Read the model definition and answer for the solid it produces. Units are mm, in the model's axes. A direction names the side the tool comes from. Give positions to 0.01 mm unless a question says otherwise; leave off trailing zeros. Loops run counter-clockwise (first coordinate to the right, second up) from the corner with the lowest first, then second, coordinate; pieces in that order, holes last. Notation, with made-up numbers: (-28, 60) -> (-20, 60) arc R24 cw to (-20, 75) -> close; hole circle Ø9 at (-6, 64.5). An arc over 180 degrees is marked (long way). One line per item, written item: value. Start each with the question number.
from build123d import *

# Parameters (mm, degrees)
SZKIC1_W                    = 33
SZKIC1_H                    = 20
DODANIE_WYCI_GNI_CIE1_DEPTH = 6
SZKIC2_W                    = 9.7
SZKIC2_H                    = 16
WYTNIJ_WYCI_GNI_CIE1_DEPTH  = 5
SZKIC2_4_W                  = 6.5
SZKIC2_4_H                  = 16
WYTNIJ_WYCI_GNI_CIE2_DEPTH  = 21.205197351
SZKIC3_W                    = 15.9
SZKIC3_H                    = 27
DODANIE_WYCI_GNI_CIE2_DEPTH = 4
SZKIC4_W                    = 10.5
SZKIC4_H                    = 23.5
WYTNIJ_WYCI_GNI_CIE3_DEPTH  = 2.5


with BuildPart() as part:
    # Szkic1 → Dodanie-wyciągnięcie1 (new body)
    with BuildSketch(Plane(origin=(0, 0, 0), x_dir=(1, 0, 0), z_dir=(0, 1, 0))):
        Rectangle(SZKIC1_W, SZKIC1_H)
    extrude(amount=DODANIE_WYCI_GNI_CIE1_DEPTH)

    # Szkic2 → Wytnij-wyciągnięcie1 (cut)
    with BuildSketch(Plane(origin=(0, 6, 0), x_dir=(1, 0, 0), z_dir=(0, 1, 0))):
        with Locations((-9.6, 0)):
            Rectangle(SZKIC2_W, SZKIC2_H)
        with Locations((9.6, 0)):
            Rectangle(SZKIC2_W, SZKIC2_H)
    extrude(amount=-WYTNIJ_WYCI_GNI_CIE1_DEPTH, mode=Mode.SUBTRACT)

    # Szkic2<4> → Wytnij-wyciągnięcie2 (cut, through all)
    with BuildSketch(Plane(origin=(0, 6, 0), x_dir=(1, 0, 0), z_dir=(0, 1, 0))):
        with Locations((-11.2, 0)):
            Rectangle(SZKIC2_4_W, SZKIC2_4_H)
        with Locations((11.2, 0)):
            Rectangle(SZKIC2_4_W, SZKIC2_4_H)
    extrude(amount=-WYTNIJ_WYCI_GNI_CIE2_DEPTH, mode=Mode.SUBTRACT)

    # Szkic3 → Dodanie-wyciągnięcie2 (add)
    with BuildSketch(Plane.XZ):
        Rectangle(SZKIC3_W, SZKIC3_H)
    extrude(amount=DODANIE_WYCI_GNI_CIE2_DEPTH)

    # Szkic4 → Wytnij-wyciągnięcie3 (cut)
    with BuildSketch(Plane.XZ.offset(4)):
        Rectangle(SZKIC4_W, SZKIC4_H)
    extrude(amount=-WYTNIJ_WYCI_GNI_CIE3_DEPTH, mode=Mode.SUBTRACT)


solid = part.part
Item 1: Consider L1, parallel to X at y = 5.25, z = -6.5; L2, parallel to X at y = -1.75, z = -8.25; L3, parallel to Z at x = -10.5, y = 1. Determine where each line is inside the solid, lowest interval first. Write a range as [from, to].
Item 2: For faces 1 (the flat face through (0, -1.5, 0)), 2 (the flat face through (15, 0, 0)), 3 (the flat face through (0, 3, -10)), 4 (the flat face through (-6, 1, 0)), 5 (the flat face through (14.45, 3, 0)), determine the directions among +Z, -Z, +X, -X, +Y, -Y from which every point of the face is accessible in a straight line to the end or side of a thin tool.
Item 3: Section D-D, the plane y = -2.5 is taken. Determine the outline of the cut face in (x, z), plus the area to 3 significant figures.
Item 4: Section C-C, the plane y = 2.25 is taken. Determine the outline of the cut face in (x, z).
Item 5: Section A-A, the plane z = 3.75 is taken. Determine the outline of the cut face in (x, y).
Item 6: Flat-ended cylindrical pins translate along their axes: pin 1 (5 mm diameter, centred on x = 7, y = 4.5, fed in from -Z); pin 2 (1 mm diameter, centred on x = -7, z = -2.5, fed in from +Y); pin 3 (1.8 mm diameter, centred on x = -10.5, y = 3, fed in from +Z); pin 4 (2.5 mm diameter, centred on x = -13, z = -2, fed in from -Y). Find the tip coordinate at first contact, or state that the pin passes through.
Item 7: Section B-B, the plane x = 10.5 is taken. Determine the outline of the cut face in (y, z), plus the area to 3 significant figures.
Item 8: Determine the mould class of faces 6 (the flat face through (0, 0, 12)), 7 (the flat face through (10, 3, -8)), 8 (the flat face through (-10, 3, -8)), 9 (the flat face through (16.5, 3, 0)) for opening direction X: pulls with the +X half, pulls with the -X half, needs draft (parallel to the pull), parting line crosses it, or undercut.
Computed values:
1. L1: [-16.5, -14.45], [-4.75, 4.75], [14.45, 16.5]
1. L2: [-7.95, -5.25], [5.25, 7.95]
1. L3: [-10, -8], [8, 10]
2. face 1: -Y
2. face 2: +Z, -Z, +X, -Y
2. face 3: -Z, +X, -X, +Y
2. face 4: +Y
2. face 5: +Y, -Y
3. outline: (-7.95, -13.5) -> (7.95, -13.5) -> (7.95, 13.5) -> (-7.95, 13.5) -> close; hole (-5.25, -11.75) -> (5.25, -11.75) -> (5.25, 11.75) -> (-5.25, 11.75) -> close
3. area: 183 mm²
4. outline: (-16.5, -10) -> (16.5, -10) -> (16.5, 10) -> (-16.5, 10) -> close; hole (-14.45, -8) -> (-4.75, -8) -> (-4.75, 8) -> (-14.45, 8) -> close; hole (4.75, -8) -> (14.45, -8) -> (14.45, 8) -> (4.75, 8) -> close
5. outline: (-16.5, 0) -> (-14.45, 0) -> (-14.45, 6) -> (-16.5, 6) -> close; (-7.95, -4) -> (-5.25, -4) -> (-5.25, -1.5) -> (5.25, -1.5) -> (5.25, -4) -> (7.95, -4) -> (7.95, 1) -> (4.75, 1) -> (4.75, 6) -> (-4.75, 6) -> (-4.75, 1) -> (-7.95, 1) -> close; (14.45, 0) -> (16.5, 0) -> (16.5, 6) -> (14.45, 6) -> close
6. pin 1: z = -10
6. pin 2: y = 1
6. pin 3: z = 10
6. pin 4: through
7. outline: (0, -10) -> (6, -10) -> (6, -8) -> (0, -8) -> close; (0, 8) -> (6, 8) -> (6, 10) -> (0, 10) -> close
7. area: 24.0 mm²
8. face 6: needs draft
8. face 7: undercut
8. face 8: undercut
8. face 9: pulls with the +X half
